Geometry: final body of the model. Coordinates: model frame, mm. Face numbers are marked on the shaded views. Coordinates: 2 decimals unless noted, no trailing zeros. Loops run counter-clockwise (first coordinate to the right, second up) from the corner with the lowest first, then second, coordinate; pieces in that order, holes last. Notation, with made-up numbers: (35, 22) - (86, 22) arc R20 cw to (86, 31) - close; hole circle Ø11 at (32, 30). An arc over 180 degrees is marked (long way). Return JSON: item names as keys, results as strings.
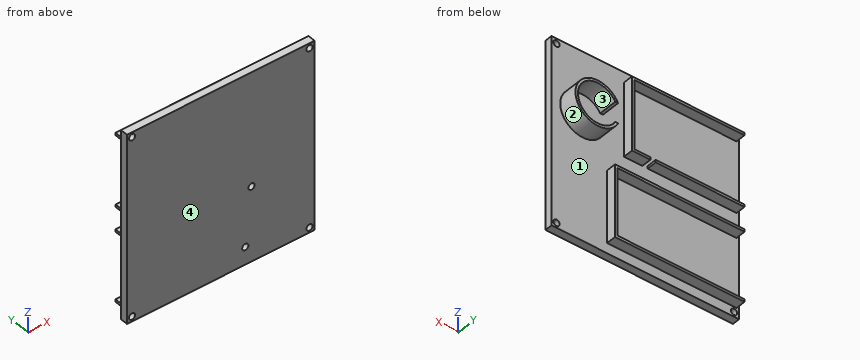
from build123d import *

# Parameters (mm, degrees)
SKETCH1_W           = 150
SKETCH1_H           = 150
BOSS_EXTRUDE1_DEPTH = 6
SKETCH2_W           = 71.08
SKETCH2_H           = 2
SKETCH2_R           = 18
SKETCH2_R_2         = 16
BOSS_EXTRUDE2_DEPTH = 7.94
SKETCH3_R           = 18
SKETCH3_R_2         = 16
BOSS_EXTRUDE3_DEPTH = 7.06
SKETCH5_R           = 2.5
CUT_EXTRUDE1_DEPTH  = 7
CUT_EXTRUDE2_DEPTH  = 15


with BuildPart() as part:
    # Sketch1 → Boss-Extrude1 (new body)
    with BuildSketch(Plane(origin=(0, 0, 0), x_dir=(1, 0, 0), z_dir=(0, 1, 0))):
        Rectangle(SKETCH1_W, SKETCH1_H)
    extrude(amount=BOSS_EXTRUDE1_DEPTH)

    # Sketch2 → Boss-Extrude2 (add)
    with BuildSketch(Plane(origin=(0, 6, 0), x_dir=(1, 0, 0), z_dir=(0, 1, 0))):
        Polygon((30.6, 67), (-73, 67), (-73, 65), (28.6, 65), (28.6, 11.5), (-73, 11.5), (-73, 9.5), (30.6, 9.5), align=None)
        with Locations((-37.46, -9.2)):
            Rectangle(SKETCH2_W, SKETCH2_H)
        Polygon((-73, -65), (-73, -67), (17, -67), (17, -8.2), (2.3, -8.2), (2.3, -10.2), (15, -10.2), (15, -65), align=None)
        with Locations((50, -25)):
            Circle(SKETCH2_R)
        with Locations((50, -25)):
            Circle(SKETCH2_R_2, mode=Mode.SUBTRACT)
    extrude(amount=BOSS_EXTRUDE2_DEPTH)

    # Sketch3 → Boss-Extrude3 (add)
    with BuildSketch(Plane(origin=(0, 13.94, 0), x_dir=(1, 0, 0), z_dir=(0, 1, 0))):
        with Locations((50, -25)):
            Circle(SKETCH3_R)
        with Locations((50, -25)):
            Circle(SKETCH3_R_2, mode=Mode.SUBTRACT)
    extrude(amount=BOSS_EXTRUDE3_DEPTH)

    # Sketch5 → Cut-Extrude1 (cut, through all)
    with BuildSketch(Plane(origin=(0, 6, 0), x_dir=(1, 0, 0), z_dir=(0, 1, 0))):
        with Locations((-71, 71)):
            Circle(SKETCH5_R)
        with Locations((19.6, 61)):
            Circle(SKETCH5_R)
        with Locations((24.6, 15.5)):
            Circle(SKETCH5_R)
        with Locations((71, 71)):
            Circle(SKETCH5_R)
        with Locations((71, -71)):
            Circle(SKETCH5_R)
        with Locations((-71, -71)):
            Circle(SKETCH5_R)
    extrude(amount=-CUT_EXTRUDE1_DEPTH, mode=Mode.SUBTRACT)

    # Sketch6 → Cut-Extrude2 (cut)
    with BuildSketch(Plane(origin=(0, 21, 0), x_dir=(1, 0, 0), z_dir=(0, 1, 0))):
        with BuildLine():
            Line((33.875484503, -33), (33.875484503, -17))
            ThreePointArc((33.875484503, -17), (32, -25), (33.875484503, -33))
        make_face()
        with BuildLine():
            ThreePointArc((36.143593539, -33), (34, -25), (36.143593539, -17))
            Line((36.143593539, -17), (33.875484503, -17))
            Line((33.875484503, -17), (33.875484503, -33))
            Line((33.875484503, -33), (36.143593539, -33))
        make_face()
    extrude(amount=-CUT_EXTRUDE2_DEPTH, mode=Mode.SUBTRACT)


solid = part.part
Item 1: Ray query, probe 1 along Z at (x, y) = (71, 3.9); probe 2 along Z at (x, y) = (-13, 10.75). Return the intervals inside material, ascending. Write a range as from..to.
Worked out:
{"probe 1": "-75..-73.5, -68.5..68.5, 73.5..75", "probe 2": "-67..-65, -11.5..-9.5, 8.2..10.2, 65..67"}
Item 2: Section query C-C, the plane z = -15.5. Return loops of the section in (x, y), and give its area (3 significant figures).
Worked out:
{"outline": "(-75, 0) - (22.1, 0) - (22.1, 6) - (-75, 6) - close; (27.1, 0) - (75, 0) - (75, 6) - (30.6, 6) - (30.6, 13.94) - (28.6, 13.94) - (28.6, 6) - (27.1, 6) - close", "area": "886 mm^2"}
Item 3: Section query B-B, the plane x = 71. Return loops of the section in (y, z), and give its area (3 significant figures).
Worked out:
{"outline": "(0, -75) - (6, -75) - (6, -73.5) - (0, -73.5) - close; (0, -68.5) - (6, -68.5) - (6, 68.5) - (0, 68.5) - close; (0, 73.5) - (6, 73.5) - (6, 75) - (0, 75) - close", "area": "840 mm^2"}
Item 4: Mould query, pull axis Z, two halves, no side actions, for the marked faces 1, 2, 3 and 4. Classes: +Z half, -Z half, draft (parallel to the pull), parting line (faces both ways), or undercut.
Worked out:
{"face 1": "undercut", "face 2": "parting line", "face 3": "undercut", "face 4": "draft"}
Item 5: Section query D-D, the plane x = 24.6. Return loops of the section in (y, z).
Worked out:
{"outline": "(0, -75) - (6, -75) - (6, -67) - (13.94, -67) - (13.94, -65) - (6, -65) - (6, -18) - (0, -18) - close; (0, -13) - (6, -13) - (6, -11.5) - (13.94, -11.5) - (13.94, -9.5) - (6, -9.5) - (6, 75) - (0, 75) - close"}
Item 6: Section query A-A, the plane z = -71. Return loops of the section in (x, y).
Worked out:
{"outline": "(-75, 0) - (-73.5, 0) - (-73.5, 6) - (-75, 6) - close; (-68.5, 0) - (68.5, 0) - (68.5, 6) - (-68.5, 6) - close; (73.5, 0) - (75, 0) - (75, 6) - (73.5, 6) - close"}
Item 7: First-contact query: pin 1 Ø1 at (y, z) = (11.5, 65.5) entering from -X; pin 2 Ø2.5 at (x, y) = (-19, 9) entering from -Z; pin 3 Ø3 at (y, z) = (8.5, -32.5) entering from -X; pin 4 Ø4.5 at (x, z) = (-71, 71) entering from -Y. Flat tips, straight axial feed; report the tip coordinate or a pass-through.
Worked out:
{"pin 1": "x = -73", "pin 2": "z = -67", "pin 3": "x = 28.6", "pin 4": "through"}
